Model file for the job. Use its own axes, mm. Round coordinates to 2 decimals unless told otherwise and drop trailing zeros. Loops run counter-clockwise (first coordinate to the right, second up) from the corner with the lowest first, then second, coordinate; pieces in that order, holes last. Notation, with made-up numbers: (-0.75, -38.75) -> (55.25, -38.75) arc R31 cw to (55.25, -5.75) -> close; hole circle Ø4 at (26, 42). An arc over 180 degrees is marked (long way). Use a Markdown table: item, result.
Autodesk Inventor part; units mm, degrees
ref_plane "YZ Plane" through (0, 0, 0) normal (1, 0, 0) x (0, 1, 0)
ref_plane "XZ Plane" through (0, 0, 0) normal (0, 1, 0) x (-1, 0, 0)
ref_plane "XY Plane" through (0, 0, 0) normal (0, 0, 1) x (1, 0, 0)
sketch "Sketch1" plane through (0, 0, 0) normal (0, 1, 0) x (-1, 0, 0)
  circle A0 centre (0, 0) radius 19.05
  circle A1 centre (0, 0) radius 11.1125
  dimension "d0" = 38.1
  dimension "d1" = 22.225
extrude "Extrusion1" add sketch "Sketch1" along normal blind 2.54
sketch "Sketch2" plane through (0, 2.54, 0) normal (0, 1, 0) x (1, 0, 0)
  line L0 (0, 0) -> (0, -14.2875)
  line L1 (0, -14.2875) -> (-13.5882, -4.4151)
  line L2 (-13.5882, -4.4151) -> (-8.398, 11.5588)
  line L3 (-8.398, 11.5588) -> (8.398, 11.5588)
  line L4 (8.398, 11.5588) -> (13.5882, -4.4151)
  line L5 (13.5882, -4.4151) -> (0, -14.2875)
  dimension "d4" = 14.2875
hole "Hole1" at (0, 2.54, 14.2875) at (-13.5882, 2.54, 4.4151) at (-8.398, 2.54, -11.5588) at (8.398, 2.54, -11.5588) at (13.5882, 2.54, 4.4151) direction (0, -1, 0) diameter 2.8956 end through all
properties part number "wheel-drill-template"
Q1. Flat gauge pin, fed straight in: pin 1 (1 mm diameter, centred on y = 0.5, z = -12.5, fed in from -X). Where does the tip first touch, or does it go through?
Results list:
| item | result |
|---|---|
| pin 1 | stops at x = -14.8 |
Q2. Drill centre lines: L1, parallel to Z at x = -1, y = 2.2; L2, parallel to X at y = 1.9, z = 5.5; L3, parallel to Z at x = 2.5, y = 2. Where is each one in solid material? Low to high. Write a range as from..to.
Results list:
| item | result |
|---|---|
| L1 | z = -19.02..-11.07, 11.07..13.24, 15.33..19.02 |
| L2 | x = -18.24..-14.55, -12.63..-9.66, 9.66..12.63, 14.55..18.24 |
| L3 | z = -18.89..-10.83, 10.83..18.89 |
Q3. Band-saw the part on A-A, the plane x = 0. Give the cut face in (y, z).
Results list:
| item | result |
|---|---|
| outline | (0, -19.05) -> (2.54, -19.05) -> (2.54, -11.11) -> (0, -11.11) -> close; (0, 11.11) -> (2.54, 11.11) -> (2.54, 12.84) -> (0, 12.84) -> close; (0, 15.74) -> (2.54, 15.74) -> (2.54, 19.05) -> (0, 19.05) -> close |
Q4. Band-saw the part on D-D, the plane x = -5. Give the cut face in (y, z).
Results list:
| item | result |
|---|---|
| outline | (0, -18.38) -> (2.54, -18.38) -> (2.54, -9.92) -> (0, -9.92) -> close; (0, 9.92) -> (2.54, 9.92) -> (2.54, 18.38) -> (0, 18.38) -> close |
Q5. Band-saw the part on B-B, the plane z = 0. Give the cut face in (x, y), plus the area to 3 significant figures.
Results list:
| item | result |
|---|---|
| outline | (-19.05, 0) -> (-11.11, 0) -> (-11.11, 2.54) -> (-19.05, 2.54) -> close; (11.11, 0) -> (19.05, 0) -> (19.05, 2.54) -> (11.11, 2.54) -> close |
| area | 40.3 mm² |
Q6. Band-saw the part on C-C, the plane z = -12. Give the cut face in (x, y).
Results list:
| item | result |
|---|---|
| outline | (-14.8, 0) -> (-9.78, 0) -> (-9.78, 2.54) -> (-14.8, 2.54) -> close; (-7.02, 0) -> (7.02, 0) -> (7.02, 2.54) -> (-7.02, 2.54) -> close; (9.78, 0) -> (14.8, 0) -> (14.8, 2.54) -> (9.78, 2.54) -> close |
Q7. Pull direction Z, two halves, no side cores. Call faces 1 (the face through (-8, 2.54, -8)), 2 (the face through (-6.985, 1.252, -11.873)), 3 (the face through (15.12, 1.25, 11.59)): released by +Z, released by -Z, zero draft, split by the parting line, or undercut.
Results list:
| item | result |
|---|---|
| face 1 | zero draft |
| face 2 | undercut |
| face 3 | split by the parting line |
